For this review, take the finished solid that the model builds, in its own axes (mm). Face numbers are marked on the shaded views. Coordinates: 2 decimals unless noted, no trailing zeros. Loops run counter-clockwise (first coordinate to the right, second up) from the corner with the lowest first, then second, coordinate; pieces in that order, holes last. Notation, with made-up numbers: M -9.5,44.5 L -4.5,44.5 A14 cw -4.5,60.5 Z; hole C -22.75,-9 d4. An arc over 180 degrees is marked long. Write each question's results on one line, items separated by ' | '. Start each with the question number.
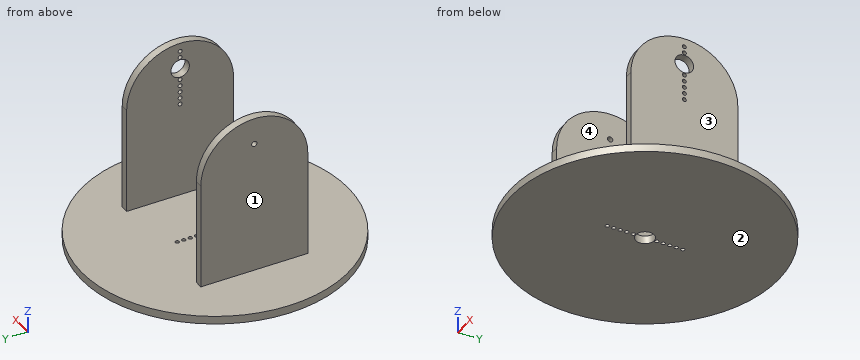
Solid Edge part; units mm, degrees
sketch "Sketch1" plane through (0, 0, 0) normal (0, 0, 1) x (1, 0, 0)
  circle A0 centre (0, 0) radius 50
extrude "Protrusion1" add sketch "Sketch1" along normal blind 3
sketch "Sketch2" plane through (0, 0, 3) normal (0, 0, 1) x (1, 0, 0)
  circle A0 centre (0, 0) radius 3.47
  circle A1 centre (0, 4.4) radius 0.74
  circle A2 centre (0, 6.83) radius 0.74
  circle A3 centre (0, 9.26) radius 0.74
  circle A4 centre (0, 11.69) radius 0.74
  circle A5 centre (0, 14.12) radius 0.74
  circle A6 centre (0, -4.4) radius 0.74
  circle A7 centre (0, -6.83) radius 0.74
  circle A8 centre (0, -9.26) radius 0.74
  circle A9 centre (0, -11.69) radius 0.74
  circle A10 centre (0, -14.12) radius 0.74
extrude "ExtrudedCutout_1" cut sketch "Sketch2" against normal blind 36.9192
sketch "Sketch3" plane through (0, 0, 3) normal (0, 0, 1) x (1, 0, 0)
  line L0 (-23.5, 20) -> (-26.5, 20)
  line L1 (-26.5, 20) -> (-26.5, -20)
  line L2 (-26.5, -20) -> (-23.5, -20)
  line L3 (-23.5, -20) -> (-23.5, 20)
  line L4 (26.5, 20) -> (23.5, 20)
  line L5 (23.5, 20) -> (23.5, -20)
  line L6 (23.5, -20) -> (26.5, -20)
  line L7 (26.5, -20) -> (26.5, 20)
extrude "ExtrudedProtrusion_2" add sketch "Sketch3" along normal blind 70
sketch "Sketch4" plane through (26.5, 0, 38) normal (1, 0, 0) x (0, 1, 0)
  arc A0 (-20, 5) -> (20, 5) centre (0, 5) cw
  line L0 (21.1932, 5) -> (20, 5)
  line L1 (21.1932, 36.3058) -> (21.1932, 5)
  line L2 (-22.4171, 36.3058) -> (21.1932, 36.3058)
  line L3 (-22.4171, 5) -> (-22.4171, 36.3058)
  line L4 (-20, 5) -> (-22.4171, 5)
extrude "ExtrudedCutout_2" cut sketch "Sketch4" against normal blind 67.3152
sketch "Sketch5" plane through (26.5, 0, 33) normal (1, 0, 0) x (0, 1, 0)
  circle A0 centre (0, 20) radius 3.47
  circle A1 centre (0, 24.4) radius 0.725
  circle A2 centre (0, 26.83) radius 0.725
  circle A3 centre (0, 15.6) radius 0.725
  circle A4 centre (0, 13.17) radius 0.725
  circle A5 centre (0, 10.74) radius 0.725
  circle A6 centre (0, 8.31) radius 0.725
  circle A7 centre (0, 5.88) radius 0.725
extrude "ExtrudedCutout_3" cut sketch "Sketch5" against normal blind 3
sketch "Sketch6" plane through (26.5, 0, 33) normal (1, 0, 0) x (0, 1, 0)
  circle A0 centre (0, 24.4) radius 0.74
  circle A1 centre (0, 26.83) radius 0.74
  circle A2 centre (0, 5.88) radius 0.74
  circle A3 centre (0, 8.325) radius 0.74
  circle A4 centre (0, 10.74) radius 0.74
  circle A5 centre (0, 13.17) radius 0.74
  circle A6 centre (0, 15.6) radius 0.74
extrude "Cutout1" cut sketch "Sketch6" against normal blind 3
sketch "Sketch7" plane through (-26.5, 0, 33) normal (-1, 0, 0) x (0, 1, 0)
  circle A0 centre (0, -20) radius 1
extrude "Cutout2" cut sketch "Sketch7" against normal blind 4.0137
Q1. The part is to be moulded in two halves that separate along X. For the marked faces 1, 2, 3 and 4, say which applies: pulls with the +X half, pulls with the -X half, needs draft (parallel to the pull), parting line crosses it, or undercut.
Q2. Take a section at C-C, the plane y = 30. Give the boundary of the cut face in (x, z).
Q3. Insertion check: P1, Ø1, axis at x = 16.5, y = -0.5, coming from the +Z side; P2, Ø2.5, axis at x = 25, z = 18.5, coming from the -Y side; P3, Ø1.7, axis at y = 0, z = 48.6, coming from the -X side. Each pin has a flat end and moves straight along its axis. Give the tip position at first contact, or say it passes through.
Q4. Take a section at B-B, the plane x = 10. Give the boundary of the cut face in (y, z), then the cut area to 3 significant figures.
Q5. Take a section at A-A, the plane z = 9.5. Give the boundary of the cut face in (x, y), then the cut area to 3 significant figures.
Q6. To check wall thickness, follow line 1 along X through (y, z) = (2.5, 21); line 2 along Z through (x, y) = (8.5, -20.5); line 3 along Y through (x, z) = (-25.5, 39). State the ranges of each line that lie inside material, in increasing order.
Results:
1) face 1: pulls with the -X half | face 2: needs draft | face 3: pulls with the +X half | face 4: undercut
2) outline: M -40,0 L 40,0 L 40,3 L -40,3 Z
3) P1: z = 3 | P2: y = -20 | P3: x = -26.5
4) outline: M -48.99,0 L 48.99,0 L 48.99,3 L -48.99,3 Z | area: 294 mm^2
5) outline: M -26.5,-20 L -23.5,-20 L -23.5,20 L -26.5,20 Z; M 23.5,-20 L 26.5,-20 L 26.5,20 L 23.5,20 Z | area: 240 mm^2
6) line 1: -26.5 to -23.5, 23.5 to 26.5 | line 2: 0 to 3 | line 3: -20 to 20
